The listing builds one solid part. Answer for the finished solid, in the listing's coordinates (mm). Round coordinates to 2 decimals unless told otherwise and drop trailing zeros. Order: outer loops, then holes, each group sorted by start corner. A loop starts at its lowest first (then second) coordinate and runs counter-clockwise, first axis right, second up. Notation, with made-up numbers: (1, 50.25) - (21, 50.25) arc R20 cw to (21, 77.25) - close; hole circle Ø4 at (61.5, 35). An arc over 180 degrees is marked (long way). Use CSV: the item, a comma, the result in double quotes. Start each with the question number.
Item 1: Find section C-C, the plane z = -1.95. Give the vertices of the cut face in (x, y) (3 decimals).
Item 2: Straight lines are drawn through the part: line 1 along Y through (x, z) = (0, 0.65); line 2 along Z through (x, y) = (-123.5, -16.5); line 3 along Z through (x, y) = (-133, -8.25). For each, find the intervals that lie inside material, in ascending order. Write a range as [from, to].
Item 3: Find section B-B, the plane y = 5. Give the vertices of the cut face in (x, z) (3 decimals).
Item 4: Flat-ended cylindrical pins translate along their axes: P1, Ø4.5, axis at x = 0, y = -5, coming from the -Z side; P2, Ø1.5, axis at x = -31, z = -1, coming from the +Y side; P3, Ø5, axis at x = -142.5, y = -5, coming from the -Z side; P4, Ø8.5, axis at x = 152.325, y = -5, coming from the +Z side. Find the tip coordinate at first contact, or state that the pin passes through.
Item 5: Find section A-A, the plane x = 61. Give the vertices of the cut face in (y, z), plus the area to 3 significant figures.
```python
from build123d import *

# Parameters (mm, degrees)
SKETCH_1_W               = 357.45
SKETCH_1_H               = 18
EXTRUDE_1_DEPTH          = 0.8
SKETCH_8_R               = 2.6
CUT_EXTRUDE_1_DEPTH      = 179.953249831
SM_START                 = -178.725
SM_EDGE_FLANGE_1_DEPTH   = 357.45
SM_EDGE_FLANGE_1_2_DEPTH = 357.45
SKETCH_12_R              = 2.6
CUT_EXTRUDE_2_DEPTH      = 10


# Read off the part's stored shape, not the designer's step: Ребро-кромка1
with BuildPart() as part:
    # Sketch 1 → Вытянуть1 (new body)
    with BuildSketch(Plane.XY):
        Rectangle(SKETCH_1_W, SKETCH_1_H)
    extrude(amount=EXTRUDE_1_DEPTH)

    # Эскиз8 → Вырез-Вытянуть1 (cut, through all)
    with BuildSketch(Plane.XY.offset(0.8)):
        with Locations((152.325, -5)):
            Circle(SKETCH_8_R)
        with Locations((-152.325, -5)):
            Circle(SKETCH_8_R)
    extrude(amount=-CUT_EXTRUDE_1_DEPTH, mode=Mode.SUBTRACT)

    # Ребро-кромка1 outline → Ребро-кромка1 (cut)
    with BuildSketch(Plane.YZ.offset(SM_START)):
        with BuildLine():
            Line((-9, 0.8), (-9, 0.786295462))
            ThreePointArc((-9, 0.786295462), (-8.889364261, 0.796570599), (-8.778305337, 0.8))
            Line((-8.778305337, 0.8), (-9, 0.8))
        make_face()
    extrude(amount=SM_EDGE_FLANGE_1_DEPTH, mode=Mode.SUBTRACT)

    # Sm Edge Flange 1 2 outline → Sm Edge Flange 1 2 (add)
    with BuildSketch(Plane.YZ.offset(SM_START)):
        with BuildLine():
            ThreePointArc((-9, 0.786295462), (-9.275580767, 0.729947152), (-9.539018208, 0.631354017))
            Line((-9.539018208, 0.631354017), (-18.2404336, -3.426182617))
            Line((-18.2404336, -3.426182617), (-17.902338991, -4.151228847))
            Line((-17.902338991, -4.151228847), (-9.200923599, -0.093692213))
            ThreePointArc((-9.200923599, -0.093692213), (-8.994744951, -0.023703993), (-8.778305337, 0))
            Line((-8.778305337, 0), (-9, 0))
            Line((-9, 0), (-9, 0.786295462))
        make_face()
    extrude(amount=SM_EDGE_FLANGE_1_2_DEPTH)

    # Эскиз12 → Вырез-Вытянуть2 (cut)
    with BuildSketch(Plane.XY.offset(0.8)):
        with Locations((0, -5)):
            Circle(SKETCH_12_R)
    extrude(amount=-CUT_EXTRUDE_2_DEPTH, mode=Mode.SUBTRACT)


solid = part.part
```
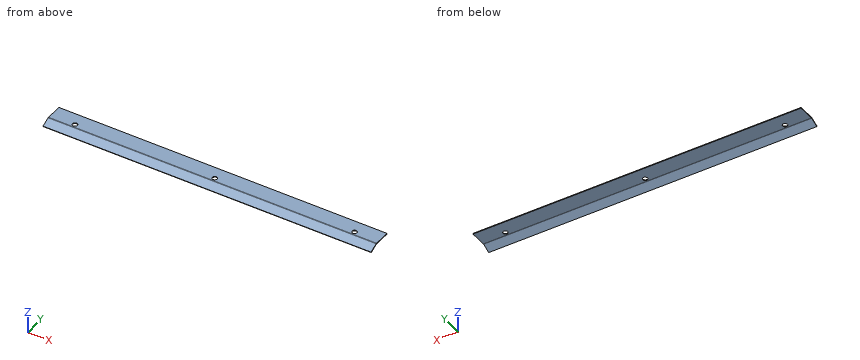
Worked out:
1,outline,"(-178.725, -15.075) - (178.725, -15.075) - (178.725, -13.182) - (-178.725, -13.182) - close"
2,line 1,"y = [-9.5, -7.6], [-2.4, 9]"
2,line 2,"z = [-3.5, -2.61]"
2,line 3,"z = [0, 0.8]"
3,outline,"(-178.725, 0) - (178.725, 0) - (178.725, 0.8) - (-178.725, 0.8) - close"
4,P1,"passes through"
4,P2,"stops at y = -9.54"
4,P3,"stops at z = 0"
4,P4,"stops at z = 0.8"
5,outline,"(-18.24, -3.43) - (-17.9, -4.15) - (-9.2, -0.09) arc R1 cw to (-8.78, 0) - (9, 0) - (9, 0.8) - (-8.78, 0.8) arc R1.8 ccw to (-9.54, 0.63) - close"
5,area,"22.4 mm²"
